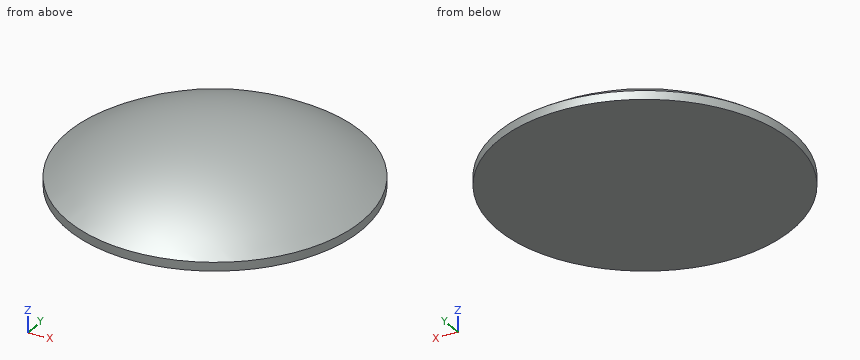
```python
from build123d import *

# Parameters (mm, degrees)
SKETCH2_OUTSIDE_W  = 117.086
SKETCH2_OUTSIDE_H  = 117.086
SKETCH2_OUTSIDE_R  = 25.4
CUT_EXTRUDE1_DEPTH = 86.476
SKETCH3_R          = 25.4
CUT_EXTRUDE2_DEPTH = 76.606


with BuildPart() as part:
    # Sketch1 → Revolve1 (revolve)
    with BuildSketch(Plane.XY):
        with BuildLine():
            Line((0, 42.738), (0, -42.738))
            ThreePointArc((0, -42.738), (-42.738, 0), (0, 42.738))
        make_face()
    revolve(axis=Axis((0, 42.738, 0), (0, -1, 0)))

    # Sketch2 outside → Cut-Extrude1 (cut, through all)
    with BuildSketch(Plane.XY.offset(42.738)):
        Rectangle(SKETCH2_OUTSIDE_W, SKETCH2_OUTSIDE_H)
        Circle(SKETCH2_OUTSIDE_R, mode=Mode.SUBTRACT)
    extrude(amount=-CUT_EXTRUDE1_DEPTH, mode=Mode.SUBTRACT)

    # Sketch3 → Cut-Extrude2 (cut, through all)
    with BuildSketch(Plane.XY.offset(32.868)):
        Circle(SKETCH3_R)
    extrude(amount=-CUT_EXTRUDE2_DEPTH, mode=Mode.SUBTRACT)


solid = part.part
```
For this review, take the finished solid that the model builds, in its own axes (mm). Give positions to 0.01 mm unless a question says otherwise; leave off trailing zeros. Write each loop counter-clockwise with the first axis right and the second up, starting at its lowest first coordinate (ties: lowest second). Pieces come first, ordered by that corner, then holes. Notation, with made-up numbers: M 32.5,-17 L 63.5,-17 A17 cw 63.5,-5 Z; hole C 82.5,-27 d10. An arc over 180 degrees is marked long. Answer as a JSON object with one key per item and string values. Group by question number.
Item 1: For probe 1 along Y at (x, z) = (-5, 39); probe 2 along Z at (x, y) = (-16, 6.5); probe 3 along Z at (x, y) = (-6.5, 16.5), list the stretches that pass through material, from the lowest coordinate up. Write a range as [from, to].
Item 2: Consider section D-D on z = 40.75. Write out the cut boundary in (x, y), plus the area to 3 significant figures.
Item 3: Consider section A-A on y = 0. Write out the cut boundary in (x, z).
Item 4: For pin 1 Ø10 at (x, y) = (13, -2) entering from +Z; pin 2 Ø4 at (y, z) = (-2, 41) entering from +X; pin 3 Ø3 at (y, z) = (9, 36) entering from +X, all flat-tipped, find the tip position at first contact; note any pin that passes through.
Item 5: Consider section C-C on z = 33.5. Write out the cut boundary in (x, y), plus the area to 3 significant figures.
Check result:
{
 "1": {"probe 1": "y = [-16.75, 16.75]", "probe 2": "z = [32.87, 39.09]", "probe 3": "z = [32.87, 38.88]"},
 "2": {"outline": "C 0,0 d25.77", "area": "521 mm^2"},
 "3": {"outline": "M -25.4,32.87 L 25.4,32.87 L 25.4,34.37 A42.74 ccw -25.4,34.37 Z"},
 "4": {"pin 1": "stops at z = 41.95", "pin 2": "stops at x = 17.37", "pin 3": "stops at x = 23.63"},
 "5": {"outline": "C 0,0 d50.8", "area": "2,030 mm^2"}
}
